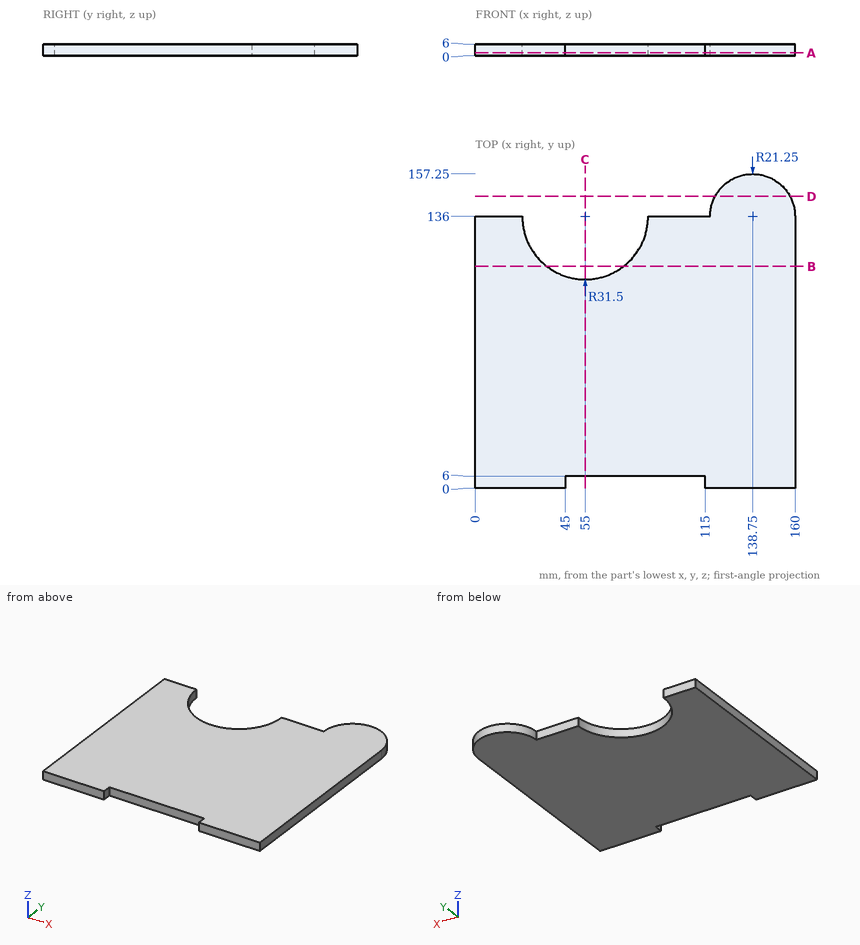
Input: dimensioned drawing with shaded views. Units: mm. Origin: part minimum x, y, z. Give positions to 0.01 mm unless a question says otherwise; leave off trailing zeros. Write each loop counter-clockwise with the first axis right and the second up, starting at its lowest first coordinate (ties: lowest second). Pieces come first, ordered by that corner, then holes. Notation, with made-up numbers: M 38,71.25 L 96,71.25 A16 cw 96,94.25 Z; hole C 18,-6.75 d5. An arc over 180 degrees is marked long. Return JSON: item names as keys, results as strings. Group by question number.
1) Cut plane C-C, the plane x = 55. Output: boundary loops of the cut face in (y, z), plus the area to 3 significant figures.
2) Cut plane A-A, the plane z = 1.55. Output: boundary loops of the cut face in (x, y).
3) Cut plane D-D, the plane y = 146. Output: boundary loops of the cut face in (x, z), plus the area to 3 significant figures.
4) Cut plane B-B, the plane y = 111. Output: boundary loops of the cut face in (x, z), plus the area to 3 significant figures.
5) Material intervals for line 1 along Y through (x, z) = (99.5, 0.95); line 2 along Y through (x, z) = (16, 2.55); line 3 along X through (y, z) = (114.5, 4.3), sorted ascending. Write a range as [from, to].
6) Pin query (flat end, axial travel): P1, Ø3, axis at x = 97.5, z = 2, coming from the +Y side. Return the tip coordinate at first contact, or that it passes through.
Recorded:
{
 "1": {"outline": "M 6,0 L 104.5,0 L 104.5,6 L 6,6 Z", "area": "591 mm²"},
 "2": {"outline": "M 0,0 L 45,0 L 45,6 L 115,6 L 115,0 L 160,0 L 160,136 A21.25 ccw 117.5,136 L 86.5,136 A31.5 cw 23.5,136 L 0,136 Z"},
 "3": {"outline": "M 120,0 L 157.5,0 L 157.5,6 L 120,6 Z", "area": "225 mm²"},
 "4": {"outline": "M 0,0 L 35.84,0 L 35.84,6 L 0,6 Z; M 74.16,0 L 160,0 L 160,6 L 74.16,6 Z", "area": "730 mm²"},
 "5": {"line 1": "y = [6, 136]", "line 2": "y = [0, 136]", "line 3": "x = [0, 31.98], [78.02, 160]"},
 "6": {"P1": "stops at y = 136"}
}
